The model under review builds one solid part; all positions refer to its coordinate system, in mm. A direction names the side the tool comes from. Round coordinates to 2 decimals unless told otherwise and drop trailing zeros. Order: outer loops, then holes, each group sorted by start corner. A loop starts at its lowest first (then second) coordinate and runs counter-clockwise, first axis right, second up.
```python
from build123d import *

# Parameters (mm, degrees)
SKETCH_R     = 40.2
SKETCH_R_2   = 20
PAD_DEPTH    = 5
PAD001_DEPTH = 74
POCKET_DEPTH = 5
FILLET_R     = 1.5
FILLET001_R  = 7.9
SKETCH003_R  = 1.8
HOLE_DEPTH   = 5
CHAMFER_SIZE = 0.4


with BuildPart() as part:
    # Sketch → Pad (new body)
    with BuildSketch(Plane.XY):
        Circle(SKETCH_R)
        Circle(SKETCH_R_2, mode=Mode.SUBTRACT)
    extrude(amount=PAD_DEPTH)

    # Sketch001 → Pad001 (join)
    with BuildSketch(Plane.XY):
        with BuildLine():
            ThreePointArc((0, 29.5), (-29.5, 0), (0, -29.5))
            Line((0, -20), (0, -29.5))
            ThreePointArc((0, 20), (-20, 0), (0, -20))
            Line((0, 29.5), (0, 20))
        make_face()
    extrude(amount=PAD001_DEPTH)

    # Sketch002 → Pocket (cut)
    with BuildSketch(Plane.XY):
        with BuildLine():
            ThreePointArc((0, -30), (30, 0), (0, 30))
            Line((0, 30), (0, 20))
            ThreePointArc((0, -20), (20, 0), (0, 20))
            Line((0, -20), (0, -30))
        make_face()
    extrude(amount=POCKET_DEPTH, mode=Mode.SUBTRACT)

    # Fillet
    fillet_edges = [part.edges().sort_by_distance(p)[0] for p in [
        (0, -29.5, 39.5),
        (0, 29.5, 39.5),
    ]]
    fillet(fillet_edges, radius=FILLET_R)

    # Fillet001
    fillet001_edges = [part.edges().sort_by_distance(p)[0] for p in [
        (-20, 0, 74),
        (0, -20, 39.5),
        (0, 20, 39.5),
    ]]
    fillet(fillet001_edges, radius=FILLET001_R)

    # Sketch003 → Hole (cut)
    with BuildSketch(Plane.XY):
        with Locations((-36.6, 0)):
            Circle(SKETCH003_R)
        with Locations((18.3, 31.69653)):
            Circle(SKETCH003_R)
        with Locations((18.3, -31.69653)):
            Circle(SKETCH003_R)
    extrude(amount=HOLE_DEPTH, mode=Mode.SUBTRACT)

    # Chamfer
    chamfer_edges = [part.edges().sort_by_distance(p)[0] for p in [
        (-40.2, 0, 5),
        (20.1, -31.69653, 5),
        (20.1, 31.69653, 5),
        (30, 0, 5),
        (-40.2, 0, 0),
        (30, 0, 0),
        (20.1, -31.69653, 0),
        (20.1, 31.69653, 0),
        (-34.8, 0, 0),
        (0, -29.75, 0),
        (0, -28.129088, 0),
        (-1.572218, -22.02857, 0),
        (-20, 0, 0),
        (-1.572218, 22.02857, 0),
        (0, 29.75, 0),
        (0, 28.129088, 0),
        (-34.8, 0, 5),
    ]]
    chamfer(chamfer_edges, length=CHAMFER_SIZE)


solid = part.part
```
(1) Consider section A-A (y = 0). Write out the cut boundary in (x, z), and give its area (3 significant figures).
Data:
outline: (-40.2, 0.4) - (-39.8, 0) - (-38.8, 0) - (-38.4, 0.4) - (-38.4, 4.6) - (-38.8, 5) - (-39.8, 5) - (-40.2, 4.6) - close; (-34.8, 0.4) - (-34.4, 0) - (-20.4, 0) - (-20, 0.4) - (-20, 66.1) arc R7.9 ccw to (-27.9, 74) - (-29.5, 74) - (-29.5, 5) - (-34.4, 5) - (-34.8, 4.6) - close; (30, 0.4) - (30.4, 0) - (39.8, 0) - (40.2, 0.4) - (40.2, 4.6) - (39.8, 5) - (30.4, 5) - (30, 4.6) - close
area: 775 mm2
(2) Draft analysis for pull direction Y (two halves, no side actions). For faces 1 (the cylindrical face through (-1.53, 22.086, 37.673)), 2 (the flat face through (-28, -2, 74)), 3 (the cylindrical face through (-29.493, 0.627, 39.017)), state which applies: pulls with the +Y half, pulls with the -Y half, needs draft (parallel to the pull), parting line crosses it, or undercut.
Data:
face 1: undercut
face 2: needs draft
face 3: parting line crosses it
(3) For faces 4 (the flat face through (-18, -17, 0)), 5 (the cylindrical face through (29.993, -0.66, 2.471)), list the 3-axis set-ups (+Z, -Z, +X, -X, +Y, -Y) from which the entire face can be reached by the end or side of a thin tool; tool diameter is ignored.
Data:
face 4: -Z, +X, -X, +Y, -Y
face 5: +Z, -Z
(4) Insertion check: pin 1 (4 mm diameter, centred on y = 29, z = 32.5, fed in from +X); pin 2 (2 mm diameter, centred on x = -14, z = 34.5, fed in from +Y); pin 3 (3 mm diameter, centred on x = -1, z = 13, fed in from +Y); pin 4 (3 mm diameter, centred on x = 18.3, y = -31.7, fed in from -Z) (1 decimal). Each pin has a flat end and moves straight along its axis. Give the tip position at first contact, or say it passes through.
Data:
pin 1: stops at x = 0
pin 2: stops at y = 26.48
pin 3: stops at y = 29.46
pin 4: passes through
(5) To check wall thickness, follow probe 1 along Y at (x, z) = (18.3, 2.75); probe 2 along Z at (x, y) = (-17.5, 26); probe 3 along Z at (x, y) = (-17, 22). State the ranges of each line that lie inside material, in increasing order.
Data:
probe 1: y = -35.79 to -33.5, -29.9 to -23.77, 23.77 to 29.9, 33.5 to 35.79
probe 2: z = 0 to 5
probe 3: z = 0 to 74
(6) Consider section B-B (z = 43.5). Write out the cut boundary in (x, y), and give its area (3 significant figures).
Data:
outline: (-5.66, -19.18) arc R20 cw to (-5.66, 19.18) arc R7.9 ccw to (0, 26.76) - (0, 27.96) arc R1.5 ccw to (-1.58, 29.46) arc R29.5 ccw to (-1.58, -29.46) arc R1.5 ccw to (0, -27.96) - (0, -26.76) arc R7.9 ccw to start
area: 721 mm2
